Part print with two shaded views. Sizes in mm from the minimum x, y, z corner. Give positions to 0.01 mm unless a question says otherwise; leave off trailing zeros. Loops run counter-clockwise (first coordinate to the right, second up) from the corner with the lowest first, then second, coordinate; pieces in that order, holes last. Notation, with made-up numbers: M -38.5,18 L 20.5,18 A10 cw 20.5,23 Z; hole C -22,41 d2. An arc over 180 degrees is marked long. Answer as a JSON object with one key per item and string values. Group by question number.
1. Slice it at B-B (z = 4.1). List the corners of the cut face in (x, y).
2. Slice it at C-C (x = 3.85). List the corners of the cut face in (y, z).
3. Drop flat-ended pins along their axis: pin 1 Ø1 at (y, z) = (194.5, 3.5) entering from -X; pin 2 Ø3 at (y, z) = (120, 0.5) entering from +X. Give the stop position or say it passes through.
4. Slice it at A-A (y = 86.5). List the corners of the cut face in (x, z).
5. Drill centre lines: line 1 along Z through (x, y) = (3.5, 236); line 2 along X through (y, z) = (100.5, 3.15); line 3 along Z through (x, y) = (5.5, 64.5). Where is each one in solid material? Low to high. Write a range as [from, to].
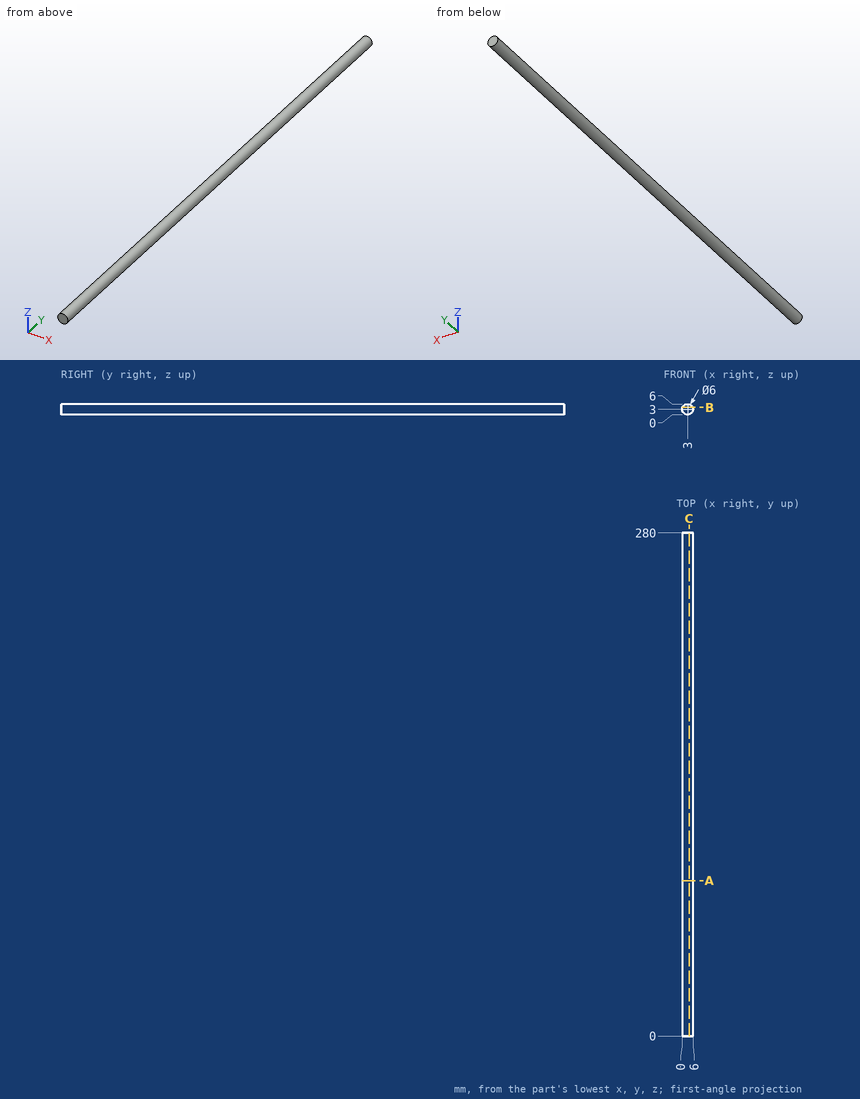
Established:
{
 "1": {"outline": "M 0.21,0 L 5.79,0 L 5.79,280 L 0.21,280 Z"},
 "2": {"outline": "M 0,0.12 L 280,0.12 L 280,5.88 L 0,5.88 Z"},
 "3": {"pin 1": "stops at x = 0", "pin 2": "stops at x = 5.83"},
 "4": {"outline": "C 3,3 d6"},
 "5": {"line 1": "z = [0.04, 5.96]", "line 2": "x = [0, 6]", "line 3": "z = [1.34, 4.66]"}
}
